Work out the finished part from the listing and answer in its coordinate system (mm). A direction names the side the tool comes from. Round coordinates to 2 decimals unless told otherwise and drop trailing zeros. Use one line per item in the form item = value.
```python
from build123d import *

# Parameters (mm, degrees)
SKETCH1_W             = 25.4
SKETCH1_H             = 25.4
SKETCH1_W_2           = 23.4
SKETCH1_H_2           = 23.4
BOSS_EXTRUDE1_DEPTH   = 304.8
BOSS_EXTRUDE1_2_DEPTH = 304.8
BOSS_EXTRUDE1_3_DEPTH = 304.8
BOSS_EXTRUDE1_4_DEPTH = 304.8
SKETCH2_W             = 25.4
SKETCH2_H             = 25.4
SKETCH2_W_2           = 23.4
SKETCH2_H_2           = 23.4
BOSS_EXTRUDE2_DEPTH   = 508
SKETCH3_W             = 25.4
SKETCH3_H             = 25.4
SKETCH3_W_2           = 23.4
SKETCH3_H_2           = 23.4
BOSS_EXTRUDE4_DEPTH   = 254
LPATTERN2_COUNT       = 2
LPATTERN2_PITCH       = 279.4


with BuildPart() as part:
    # Sketch1 → Boss-Extrude1 (new body)
    with BuildSketch(Plane(origin=(0, 0, 0), x_dir=(1, 0, 0), z_dir=(0, 1, 0))):
        with Locations((139.7, 266.7)):
            Rectangle(SKETCH1_W, SKETCH1_H)
        with Locations((139.7, 266.7)):
            Rectangle(SKETCH1_W_2, SKETCH1_H_2, mode=Mode.SUBTRACT)
    extrude(amount=BOSS_EXTRUDE1_DEPTH)



with BuildPart() as body_2:
    # Sketch1 → Boss-Extrude1 2 (new body)
    with BuildSketch(Plane(origin=(0, 0, 0), x_dir=(1, 0, 0), z_dir=(0, 1, 0))):
        with Locations((139.7, -266.7)):
            Rectangle(SKETCH1_W, SKETCH1_H)
        with Locations((139.7, -266.7)):
            Rectangle(SKETCH1_W_2, SKETCH1_H_2, mode=Mode.SUBTRACT)
    extrude(amount=BOSS_EXTRUDE1_2_DEPTH)


with BuildPart() as body_3:
    # Sketch1 → Boss-Extrude1 3 (new body)
    with BuildSketch(Plane(origin=(0, 0, 0), x_dir=(1, 0, 0), z_dir=(0, 1, 0))):
        with Locations((-139.7, -266.7)):
            Rectangle(SKETCH1_W, SKETCH1_H)
        with Locations((-139.7, -266.7)):
            Rectangle(SKETCH1_W_2, SKETCH1_H_2, mode=Mode.SUBTRACT)
    extrude(amount=BOSS_EXTRUDE1_3_DEPTH)


with BuildPart() as body_4:
    # Sketch1 → Boss-Extrude1 4 (new body)
    with BuildSketch(Plane(origin=(0, 0, 0), x_dir=(1, 0, 0), z_dir=(0, 1, 0))):
        with Locations((-139.7, 266.7)):
            Rectangle(SKETCH1_W, SKETCH1_H)
        with Locations((-139.7, 266.7)):
            Rectangle(SKETCH1_W_2, SKETCH1_H_2, mode=Mode.SUBTRACT)
    extrude(amount=BOSS_EXTRUDE1_4_DEPTH)


with BuildPart() as part_1:
    add(part.part)

    add(body_2.part)  # Boss-Extrude2 merges body 2
    # Sketch2 → Boss-Extrude2 (add)
    # profile 1 of 2: a face of its own
    with BuildSketch(Plane.XY.offset(-254)):
        with Locations((139.7, 292.1)):
            Rectangle(SKETCH2_W, SKETCH2_H)
        with Locations((139.7, 292.1)):
            Rectangle(SKETCH2_W_2, SKETCH2_H_2, mode=Mode.SUBTRACT)
    # profile 2 of 2: a face of its own
    with BuildSketch(Plane.XY.offset(-254)):
        with Locations((139.7, 12.7)):
            Rectangle(SKETCH2_W, SKETCH2_H)
        with Locations((139.7, 12.7)):
            Rectangle(SKETCH2_W_2, SKETCH2_H_2, mode=Mode.SUBTRACT)
    boss_extrude2 = extrude(amount=BOSS_EXTRUDE2_DEPTH)


    add(body_3.part)  # Boss-Extrude4 merges body 3

    add(body_4.part)  # Boss-Extrude4 merges body 4
    # Sketch3 → Boss-Extrude4 (add)
    # profile 1 of 4: a face of its own
    with BuildSketch(Plane.ZY.offset(-127)):
        with Locations((266.7, 292.1)):
            Rectangle(SKETCH3_W, SKETCH3_H)
        with Locations((266.7, 292.1)):
            Rectangle(SKETCH3_W_2, SKETCH3_H_2, mode=Mode.SUBTRACT)
    # profile 2 of 4: a face of its own
    with BuildSketch(Plane.ZY.offset(-127)):
        with Locations((-266.7, 292.1)):
            Rectangle(SKETCH3_W, SKETCH3_H)
        with Locations((-266.7, 292.1)):
            Rectangle(SKETCH3_W_2, SKETCH3_H_2, mode=Mode.SUBTRACT)
    # profile 3 of 4: a face of its own
    with BuildSketch(Plane.ZY.offset(-127)):
        with Locations((266.7, 12.7)):
            Rectangle(SKETCH3_W, SKETCH3_H)
        with Locations((266.7, 12.7)):
            Rectangle(SKETCH3_W_2, SKETCH3_H_2, mode=Mode.SUBTRACT)
    # profile 4 of 4: a face of its own
    with BuildSketch(Plane.ZY.offset(-127)):
        with Locations((-266.7, 12.7)):
            Rectangle(SKETCH3_W, SKETCH3_H)
        with Locations((-266.7, 12.7)):
            Rectangle(SKETCH3_W_2, SKETCH3_H_2, mode=Mode.SUBTRACT)
    extrude(amount=BOSS_EXTRUDE4_DEPTH)

    # LPattern2: Boss-Extrude2 ×2
    with Locations(*[(-i * LPATTERN2_PITCH, 0, 0) for i in range(1, LPATTERN2_COUNT)]):
        add(boss_extrude2)


solid = part_1.part
```
Item 1: For faces 1 (the flat face through (-127, 292, -4)), 2 (the flat face through (-140, 25.4, -4)), 3 (the flat face through (-140, 292, -254)), 4 (the flat face through (2, 25.4, 267)), determine the directions among +Z, -Z, +X, -X, +Y, -Y from which every point of the face is accessible in a straight line to the end or side of a thin tool.
Findings:
face_1 = +Y, -Y
face_2 = +X, -X
face_3 = none
face_4 = +Z, -Z
Item 2: The part is cut by section A-A, the plane z = -200.5. Give the number of separate pieces and of enclosed holes in the cut face, and give its area (3 significant figures).
Findings:
separate_pieces = 4
enclosed_holes = 4
area = 390 mm^2
Item 3: Determine the mould class of faces 5 (the flat face through (-152.4, 16, -22)), 6 (the flat face through (-136, 304.8, -1)), 7 (the flat face through (140, 151, 254)) for opening direction Y: released by +Y, released by -Y, zero draft, split by the parting line, or undercut.
Findings:
face_5 = zero draft
face_6 = released by +Y
face_7 = undercut
Item 4: Consider line 1 along Y through (x, z) = (129, 4); line 2 along X through (y, z) = (284.5, -35); line 3 along Z through (x, y) = (-29.5, 16.5). Determine where each line is inside the solid, lowest interval first.
Findings:
line_1 = 0 to 1, 24.4 to 25.4, 279.4 to 280.4, 303.8 to 304.8
line_2 = -152.4 to -151.4, -128 to -127, 127 to 128, 151.4 to 152.4
line_3 = -279.4 to -278.4, -255 to -254, 254 to 255, 278.4 to 279.4
